```python
from build123d import *

# Parameters (mm, degrees)
F0_W     = 139.7
F0_H     = 3.175
F1_DEPTH = 22.225
F4_R     = 12.7
F6_DEPTH = 3.175
F9_DEPTH = 1.5875


# Not quite as in the source:
# - a pattern or mirror of a feature is missing from the dataset's text; its kind, count and spacing are read off the source's solid


with BuildPart() as f1:
    # F0 (on Right) → F1 (new body, symmetric)
    with BuildSketch(Plane.YZ):
        with Locations((44.45, -1.5875)):
            Rectangle(F0_W, F0_H)
    extrude(amount=F1_DEPTH, both=True)

    # F2 (on Right) → F3 (revolve)
    with BuildSketch(Plane.YZ):
        with BuildLine():
            Line((0, 0), (0, 9.525))
            ThreePointArc((0, 9.525), (-11.5091012898, 7.0320228377), (-20.955, 0))
            Line((-20.955, 0), (0, 0))
        make_face()
    revolve(axis=Axis((0, 0, 4.7625), (0, 0, -1)))

    # F4
    f4_edges = [f1.edges().sort_by_distance(p)[0] for p in [
        (22.225, -25.4, -1.5875),
        (-22.225, -25.4, -1.5875),
    ]]
    fillet(f4_edges, radius=F4_R)

    # F5 (on face) → F6 (join)
    with BuildSketch(Plane(origin=(0, 114.3, 0), x_dir=(-1, 0, 0), z_dir=(0, 1, 0))):
        Polygon((-22.225, 25.4), (-22.225, 0), (22.225, 0), (22.225, 25.4), (12.7, 34.925), (12.7, 85.725), (-12.7, 85.725), (-12.7, 34.925), align=None)
    extrude(amount=-F6_DEPTH)

    # F8 (on offset) → F9 (join, symmetric)
    with BuildSketch(Plane.YZ.offset(9.525)):
        Polygon((111.125, 0), (111.125, 9.525), (85.725, 0), align=None)
    f9 = extrude(amount=F9_DEPTH, both=True)

    # F9_copies: F9 across plane
    add(f9.mirror(Plane(origin=(0, 0, 0), x_dir=(0, 0, -1), z_dir=(-1, 0, 0))))


solid = f1.part
```
Source: CAD feature listing. Evaluate the final solid. Frame: model axes, mm. A direction names the side the tool comes from. Round coordinates to 2 decimals unless told otherwise and drop trailing zeros. Write each loop counter-clockwise with the first axis right and the second up, starting at its lowest first coordinate (ties: lowest second). Pieces come first, ordered by that corner, then holes. Notation, with made-up numbers: M 69,86 L 85,86 A27 ccw 85,115 Z; hole C -6,39.5 d2. An arc over 180 degrees is marked long. Answer as a JSON object with one key per item and string values. Group by question number.
(1) Section query D-D on y = -4.5. Output: boundary loops of the cut face in (x, z) (3 decimals), then the cut area to 3 significant figures.
(2) First-contact query: pin 1 (1.6 mm diameter, centred on y = 112.5, z = 54.5, fed in from +X); pin 2 (2.5 mm diameter, centred on y = 113, z = 56, fed in from -X); pin 3 (10.5 mm diameter, centred on y = 104, z = 2.5, fed in from -X) (3 decimals); pin 4 (5 mm diameter, centred on y = 97.5, z = 5.5, fed in from -X). Flat tips, straight axial feed; report the tip coordinate or a pass-through.
(3) Section query C-C on x = -6.5. Output: boundary loops of the cut face in (y, z) (3 decimals).
(4) Section query A-A on y = 97. Output: boundary loops of the cut face in (x, z) (1 decimal), then the cut area to 3 significant figures.
(5) Section query B-B on z = 21. Output: boundary loops of the cut face in (x, y) (3 decimals).
(6) Mould query, pull axis Y, two halves, no side actions, for faces 4 (the cylindrical face through (-18.406, -21.778, -1.565)), 5 (the flat face through (-22.225, 65, -1)), 6 (the flat face through (7.938, 104, 3)). Classes: +Y half, -Y half, draft (parallel to the pull), parting line (faces both ways), or undercut.
(7) Reachability of faces 1 (the flat face through (0, 57, 0)), 2 (the flat face through (11.112, 104, 3)), 3 (the flat face through (9.55, 98.6, 4.83)) from +Z, -Z, +X, -X, +Y, -Y: full face, straight path, thin tool, end or side. Return the list, or none.
(8) Ray query, line 1 (Z direction, x = 0.5, y = 31) (3 decimals); line 2 (Y direction, x = 1, z = 28) (3 decimals); line 3 (Z direction, x = 5, y = -20) (3 decimals). Return the intervals inside material, ascending. Write a range as [from, to].
Computed values:
{
 "1": {"outline": "M -22.225,-3.175 L 22.225,-3.175 L 22.225,0 L 20.466,0 A27.447 ccw -20.466,0 L -22.225,0 Z", "area": "401 mm^2"},
 "2": {"pin 1": "x = 12.7", "pin 2": "x = -12.7", "pin 3": "x = -22.225", "pin 4": "x = -11.11"},
 "3": {"outline": "M -25.4,-3.175 L 114.3,-3.175 L 114.3,85.725 L 111.125,85.725 L 111.125,0 L 19.921,0 A27.043 ccw -19.921,0 L -25.4,0 Z"},
 "4": {"outline": "M -22.2,-3.2 L 22.2,-3.2 L 22.2,0 L 11.1,0 L 11.1,4.2 L 7.9,4.2 L 7.9,0 L -7.9,0 L -7.9,4.2 L -11.1,4.2 L -11.1,0 L -22.2,0 Z", "area": "168 mm^2"},
 "5": {"outline": "M -22.225,111.125 L 22.225,111.125 L 22.225,114.3 L -22.225,114.3 Z"},
 "6": {"face 4": "-Y half", "face 5": "draft", "face 6": "undercut"},
 "7": {"face 1": "+Z", "face 2": "+Z, +X", "face 3": "+Z, +X, -X"},
 "8": {"line 1": "[-3.175, 0]", "line 2": "[111.125, 114.3]", "line 3": "[-3.175, 0.382]"}
}
